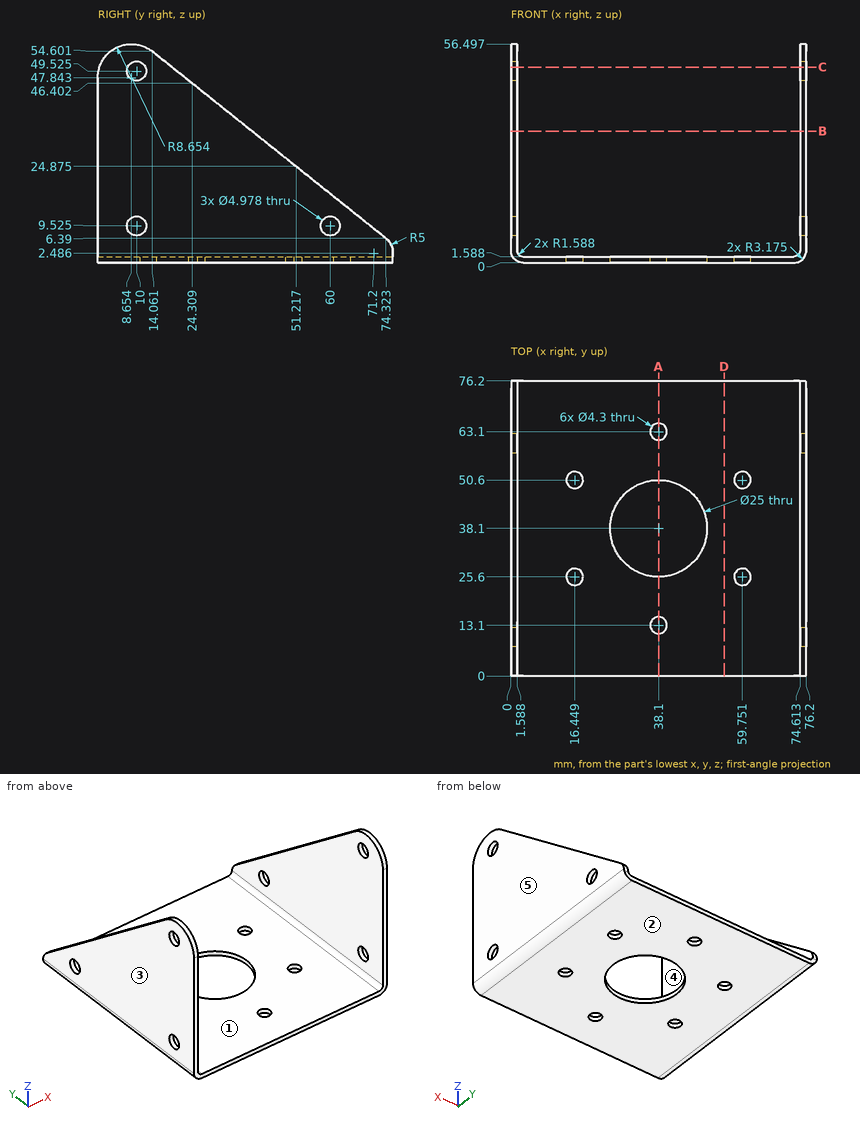
Geometry: see drawing. Coordinates: mm, zero at the bounding-box minimum. A direction names the side the tool comes from. Round coordinates to 2 decimals unless told otherwise and drop trailing zeros. Write each loop counter-clockwise with the first axis right and the second up, starting at its lowest first coordinate (ties: lowest second). Pieces come first, ordered by that corner, then holes. Notation, with made-up numbers: M 6,4.5 L 17,4.5 A18 cw 17,33.5 Z; hole C 18,48.5 d5. An arc over 180 degrees is marked long. Answer as a JSON object with one key per item and string values. Group by question number.
(1) First-contact query: pin 1 (20 mm diameter, centred on x = 38.1, y = 38.1, fed in from +Z); pin 2 (10 mm diameter, centred on x = 17, y = 25.5, fed in from -Z); pin 3 (7 mm diameter, centred on x = 59.75, y = 25.6, fed in from +Z). Flat tips, straight axial feed; report the tip coordinate or a pass-through.
(2) Reachability of the marked faces 1 and 2 from +Z, -Z, +X, -X, +Y, -Y: full face, straight path, thin tool, end or side. Return the list, or none.
(3) Section query A-A on x = 38.1. Output: boundary loops of the cut face in (y, z).
(4) Section query D-D on x = 55. Output: boundary loops of the cut face in (y, z).
(5) Ray query, line 1 (Y direction, x = 38.1, z = 1.2); line 2 (X direction, y = 7, z = 6); line 3 (Z direction, x = 63, y = 12.5). Return the intervals inside material, ascending. Write a range as [from, to].
(6) Mould query, pull axis X, two halves, no side actions, for the marked faces 3, 4 and 5. Classes: +X half, -X half, draft (parallel to the pull), parting line (faces both ways), or undercut.
(7) Section query C-C on z = 50.5. Output: boundary loops of the cut face in (x, y).
(8) Section query B-B on z = 34. Output: boundary loops of the cut face in (x, y).
Computed values:
{
 "1": {"pin 1": "through", "pin 2": "z = 0", "pin 3": "z = 1.59"},
 "2": {"face 1": "+Z, +Y, -Y", "face 2": "-Z, +X, -X, +Y, -Y"},
 "3": {"outline": "M 0,0 L 10.95,0 L 10.95,1.59 L 0,1.59 Z; M 15.25,0 L 25.6,0 L 25.6,1.59 L 15.25,1.59 Z; M 50.6,0 L 60.95,0 L 60.95,1.59 L 50.6,1.59 Z; M 65.25,0 L 76.2,0 L 76.2,1.59 L 65.25,1.59 Z"},
 "4": {"outline": "M 0,0 L 76.2,0 L 76.2,1.59 L 0,1.59 Z"},
 "5": {"line 1": "[0, 10.95], [15.25, 25.6], [50.6, 60.95], [65.25, 76.2]", "line 2": "[0, 1.59], [74.61, 76.2]", "line 3": "[0, 1.59]"},
 "6": {"face 3": "-X half", "face 4": "undercut", "face 5": "+X half"},
 "7": {"outline": "M 0,0.42 L 1.59,0.42 L 1.59,7.71 L 0,7.71 Z; M 0,12.29 L 1.59,12.29 L 1.59,19.19 L 0,19.19 Z; M 74.61,0.42 L 76.2,0.42 L 76.2,7.71 L 74.61,7.71 Z; M 74.61,12.29 L 76.2,12.29 L 76.2,19.19 L 74.61,19.19 Z"},
 "8": {"outline": "M 0,0 L 1.59,0 L 1.59,39.81 L 0,39.81 Z; M 74.61,0 L 76.2,0 L 76.2,39.81 L 74.61,39.81 Z"}
}
